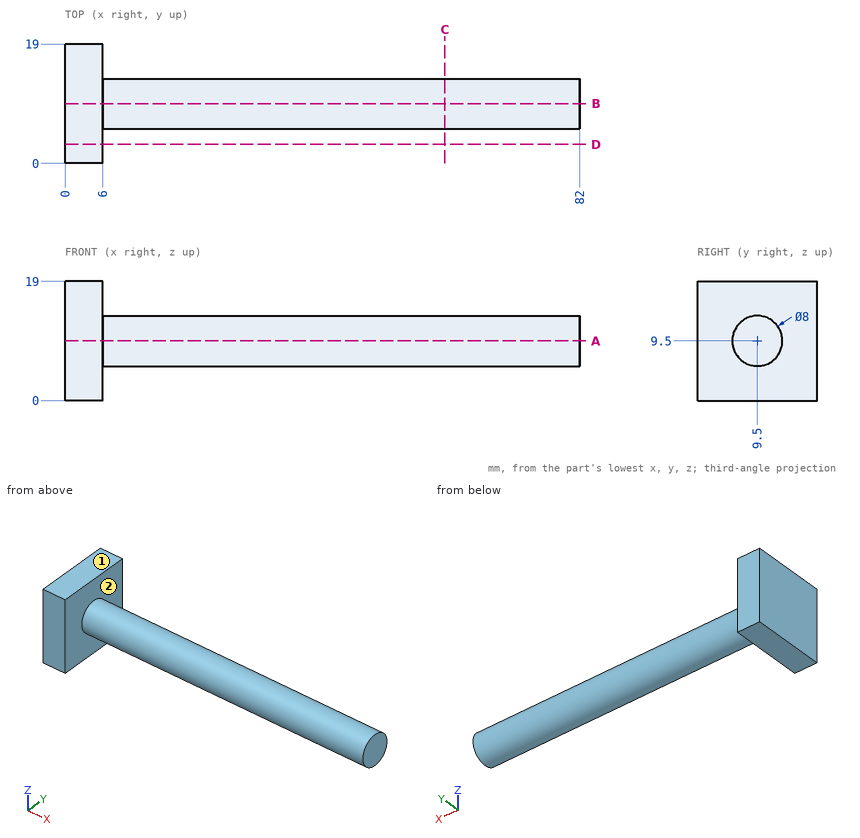
Geometry: see drawing. Coordinates: mm, zero at the bounding-box minimum. A direction names the side the tool comes from. Give positions to 0.01 mm unless a question says otherwise; leave off trailing zeros. Write each loop counter-clockwise with the first axis right and the second up, starting at its lowest first coordinate (ties: lowest second). Pieces come first, ordered by that corner, then holes. Notation, with made-up numbers: M 22.5,16.5 L 78.5,16.5 A20 ccw 78.5,22.5 Z; hole C 32.5,46.5 d2. An arc over 180 degrees is marked long. Answer in a Markdown table with one row per item. Add a question column.
(1) First-contact query: pin 1 (6 mm diameter, centred on x = 35.5, y = 4, fed in from +Z); pin 2 (8 mm diameter, centred on x = 23.5, y = 11, fed in from -Z); pin 3 (1 mm diameter, centred on x = 60.5, z = 8.5, fed in from +Y). Flat tips, straight axial feed; report the tip coordinate or a pass-through.
(2) Reachability of the marked faces 1 and 2 from +Z, -Z, +X, -X, +Y, -Y: full face, straight path, thin tool, end or side. Return the list, or none.
(3) Section C-C on x = 60.5. Return loops of the section in (y, z).
(4) Section D-D on y = 3. Return loops of the section in (x, z), and give its area (3 significant figures).
(5) Section A-A on z = 9.5. Return loops of the section in (x, y).
(6) Ray query, line 1 (X direction, y = 2, z = 17); line 2 (Y direction, x = 39.5, z = 9.25); line 3 (Z direction, x = 59.5, y = 7.5). Return the intervals inside material, ascending.
Result set:
| question | item | result |
|---|---|---|
| 1 | pin 1 | stops at z = 12.62 |
| 1 | pin 2 | stops at z = 5.5 |
| 1 | pin 3 | stops at y = 13.47 |
| 2 | face 1 | +Z, +X, -X, +Y, -Y |
| 2 | face 2 | +X |
| 3 | outline | C 9.5,9.5 d8 |
| 4 | outline | M 0,0 L 6,0 L 6,19 L 0,19 Z |
| 4 | area | 114 mm^2 |
| 5 | outline | M 0,0 L 6,0 L 6,5.5 L 82,5.5 L 82,13.5 L 6,13.5 L 6,19 L 0,19 Z |
| 6 | line 1 | x = 0 to 6 |
| 6 | line 2 | y = 5.51 to 13.49 |
| 6 | line 3 | z = 6.04 to 12.96 |
